Geometry check sheet. Reference: drawing and pictorial views, mm from the part's lowest x, y, z. A direction names the side the tool comes from. Round coordinates to 2 decimals unless told otherwise and drop trailing zeros. Order: outer loops, then holes, each group sorted by start corner. A loop starts at its lowest first (then second) coordinate and runs counter-clockwise, first axis right, second up. Notation, with made-up numbers: (-40, -10) -> (10, -10) arc R13 cw to (10, -4) -> close; hole circle Ø2 at (68.5, -39.5). An arc over 180 degrees is marked (long way). Put each result on its own line as item: value.
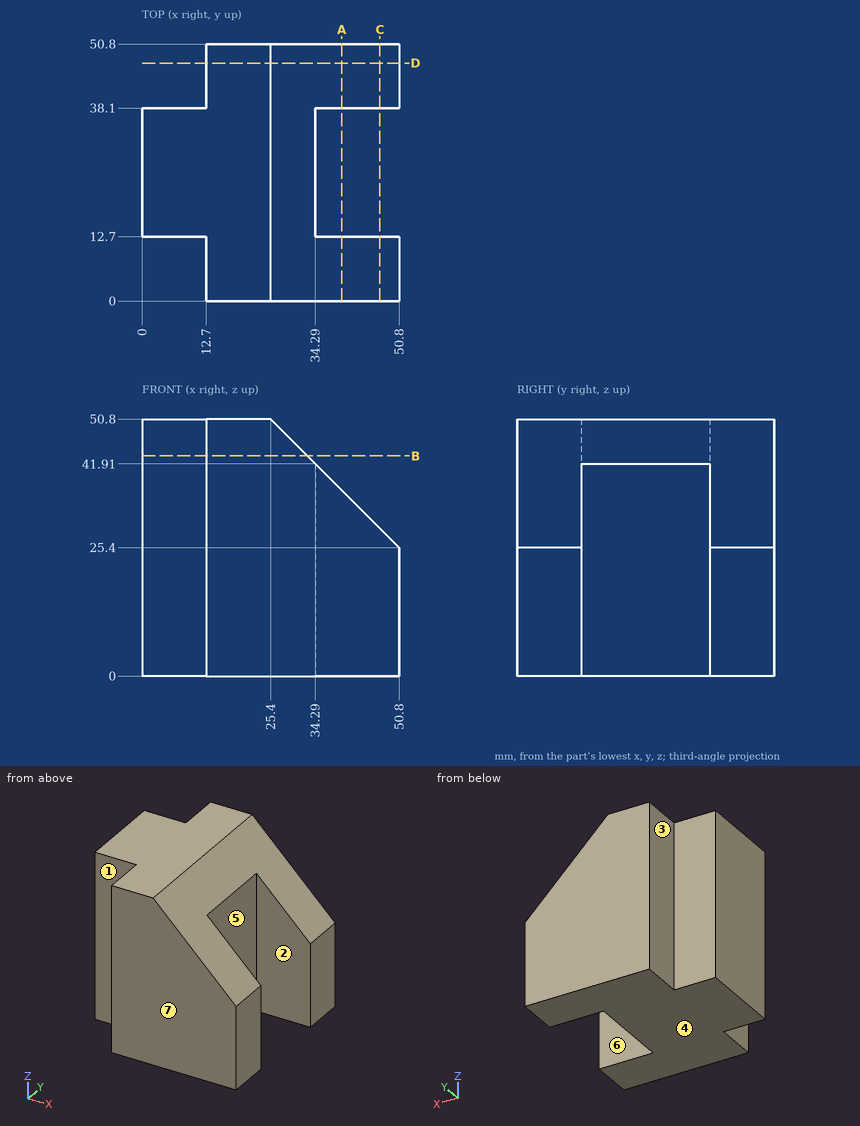
Item 1: Depth check by flat-ended pin: pin 1 Ø1.5 at (y, z) = (28, 6) entering from +X; pin 2 Ø14 at (x, z) = (5, 34.5) entering from +Y; pin 3 Ø4 at (x, z) = (5.5, 15.5) entering from -Y. Enter the tip coordinate at first touch or a pass-through.
Geometry check:
pin 1: x = 34.29
pin 2: y = 38.1
pin 3: y = 12.7
Item 2: Material ranges on line 1 along Y through (x, z) = (38, 21.5); line 2 along X through (y, z) = (39.5, 19.5); line 3 along Y through (x, z) = (10, 7), recorded low to high.
Geometry check:
line 1: 0 to 12.7, 38.1 to 50.8
line 2: 12.7 to 50.8
line 3: 12.7 to 38.1
Item 3: Sectioned sample at C-C, the plane x = 47. Record the boundary of the cut face in (y, z).
Geometry check:
outline: (0, 0) -> (12.7, 0) -> (12.7, 29.2) -> (0, 29.2) -> close; (38.1, 0) -> (50.8, 0) -> (50.8, 29.2) -> (38.1, 29.2) -> close
Item 4: Release check for a two-part mould opening along Y. For the marked faces 4, 5, 6 and 7 record: pulls with the +Y half, pulls with the -Y half, needs draft (parallel to the pull), parting line crosses it, or undercut.
Geometry check:
face 4: needs draft
face 5: undercut
face 6: undercut
face 7: pulls with the -Y half
Item 5: Tool access check on the marked faces 1, 2 and 3. Record the directions out of +Z, -Z, +X, -X, +Y, -Y that give a thin tool (end or side, any length) a straight path to the whole face; none if there is none.
Geometry check:
face 1: +Z, -Z, -X, -Y
face 2: +Z, -Z, +X
face 3: +Z, -Z, -X, +Y
Item 6: Sectioned sample at A-A, the plane x = 39.5. Record the boundary of the cut face in (y, z), then the cut area to 3 significant figures.
Geometry check:
outline: (0, 0) -> (12.7, 0) -> (12.7, 36.7) -> (0, 36.7) -> close; (38.1, 0) -> (50.8, 0) -> (50.8, 36.7) -> (38.1, 36.7) -> close
area: 932 mm2
Item 7: Sectioned sample at B-B, the plane z = 43.5. Record the boundary of the cut face in (x, y), then the cut area to 3 significant figures.
Geometry check:
outline: (0, 12.7) -> (12.7, 12.7) -> (12.7, 0) -> (32.7, 0) -> (32.7, 50.8) -> (12.7, 50.8) -> (12.7, 38.1) -> (0, 38.1) -> close
area: 1,340 mm2
Item 8: Sectioned sample at D-D, the plane y = 47. Record the boundary of the cut face in (x, z), then the cut area to 3 significant figures.
Geometry check:
outline: (12.7, 0) -> (50.8, 0) -> (50.8, 25.4) -> (25.4, 50.8) -> (12.7, 50.8) -> close
area: 1,610 mm2
